```python
from build123d import *

# Parameters (mm, degrees)
SKETCH1_W               = 89.8
SKETCH1_H               = 61.4
BOSS_EXTRUDE1_DEPTH     = 6.9
SKETCH2_R               = 2
CUT_EXTRUDE1_DEPTH      = 4
SKETCH3_W               = 97
SKETCH3_H               = 70.6
BOSS_EXTRUDE2_DEPTH     = 5
SKETCH5_W               = 10.4
SKETCH5_H               = 6.9
SKETCH5_W_2             = 3.4
BOSS_EXTRUDE3_DEPTH     = 1.8
BOSS_EXTRUDE4_START     = 1.8
SKETCH5_3_W             = 10.4
SKETCH5_3_H             = 6.9
SKETCH5_3_H_2           = 27.6
SKETCH5_3_W_2           = 3.4
BOSS_EXTRUDE4_DEPTH     = 1
BOSS_EXTRUDE6_START     = -89.8
SKETCH5_5_W             = 3.4
SKETCH5_5_H             = 6.9
SKETCH5_5_W_2           = 10.4
BOSS_EXTRUDE6_DEPTH     = 1.8
BOSS_EXTRUDE7_START     = -91.6
SKETCH5_7_W             = 3.4
SKETCH5_7_H             = 6.9
SKETCH5_7_H_2           = 27.6
SKETCH5_7_W_2           = 10.4
BOSS_EXTRUDE7_DEPTH     = 1
CUT_EXTRUDE2_DEPTH      = 120.754123102
CUT_EXTRUDE2_DEPTH_BACK = 120.754123102
SKETCH6_R               = 3.2
BOSS_EXTRUDE9_START     = -24.4
BOSS_EXTRUDE9_DEPTH     = 23.4
BOSS_EXTRUDE10_START    = -92.4
SKETCH7_4_W             = 10
SKETCH7_4_H             = 7.6
SKETCH7_4_W_2           = 4
SKETCH7_4_H_2           = 7.2
BOSS_EXTRUDE10_DEPTH    = 23.4
SKETCH9_R               = 2
CUT_EXTRUDE3_DEPTH      = 4
MIRROR4_COPY_1_SKETCH_R = 2
MIRROR4_COPY_1_DEPTH    = 4
FILLET1_R               = 5
FILLET2_R               = 5
SKETCH12_R              = 2
CUT_EXTRUDE6_DEPTH      = 4


with BuildPart() as part:
    # Sketch1 → Boss-Extrude1 (new body)
    with BuildSketch(Plane(origin=(0, 0, 0), x_dir=(1, 0, 0), z_dir=(0, 1, 0))):
        with Locations((45.3, -31.1)):
            Rectangle(SKETCH1_W, SKETCH1_H)
        Polygon((81.1, 0), (81.1, 3.6), (9.5, 3.6), (9.5, 0), (9.5, -0.4), (81.1, -0.4), align=None)
    extrude(amount=BOSS_EXTRUDE1_DEPTH)

    # Sketch2 → Cut-Extrude1 (cut)
    with BuildSketch(Plane(origin=(90.2, 0, 0), x_dir=(0, 0, -1), z_dir=(1, 0, 0))):
        with Locations((-3.45, 3.45)):
            Circle(SKETCH2_R)
    cut_extrude1 = extrude(amount=-CUT_EXTRUDE1_DEPTH, mode=Mode.SUBTRACT)

    # Mirror1: Cut-Extrude1 across plane
    add(cut_extrude1.mirror(Plane(origin=(45.3, 0, 0), x_dir=(0, 0, 1), z_dir=(1, 0, 0))), mode=Mode.SUBTRACT)

    # Sketch3 → Boss-Extrude2 (add)
    with BuildSketch(Plane(origin=(0, 0, 0), x_dir=(1, 0, 0), z_dir=(0, 1, 0))):
        with Locations((45.3, -30.1)):
            Rectangle(SKETCH3_W, SKETCH3_H)
    extrude(amount=-BOSS_EXTRUDE2_DEPTH)

    # Sketch5 → Boss-Extrude3 (add)
    with BuildSketch(Plane.ZY.offset(-0.4)):
        with Locations((30.1, 3.45)):
            Rectangle(SKETCH5_W, SKETCH5_H)
        with Locations((23.2, 3.45)):
            Rectangle(SKETCH5_W_2, SKETCH5_H)
        with Locations((37, 3.45)):
            Rectangle(SKETCH5_W_2, SKETCH5_H)
    extrude(amount=BOSS_EXTRUDE3_DEPTH)

    # Sketch5<3> → Boss-Extrude4 (add)
    with BuildSketch(Plane.ZY.offset(-0.4).offset(BOSS_EXTRUDE4_START)):
        with Locations((30.1, 3.45)):
            Rectangle(SKETCH5_3_W, SKETCH5_3_H)
        with Locations((30.1, 20.7)):
            Rectangle(SKETCH5_3_W, SKETCH5_3_H_2)
        with Locations((23.2, 20.7)):
            Rectangle(SKETCH5_3_W_2, SKETCH5_3_H_2)
        with Locations((23.2, 3.45)):
            Rectangle(SKETCH5_3_W_2, SKETCH5_3_H)
        with Locations((37, 3.45)):
            Rectangle(SKETCH5_3_W_2, SKETCH5_3_H)
        with Locations((37, 20.7)):
            Rectangle(SKETCH5_3_W_2, SKETCH5_3_H_2)
    extrude(amount=-BOSS_EXTRUDE4_DEPTH)

    # Sketch5<5> → Boss-Extrude6 (add)
    with BuildSketch(Plane.ZY.offset(-0.4).offset(BOSS_EXTRUDE6_START)):
        with Locations((23.2, 3.45)):
            Rectangle(SKETCH5_5_W, SKETCH5_5_H)
        with Locations((37, 3.45)):
            Rectangle(SKETCH5_5_W, SKETCH5_5_H)
        with Locations((30.1, 3.45)):
            Rectangle(SKETCH5_5_W_2, SKETCH5_5_H)
    extrude(amount=-BOSS_EXTRUDE6_DEPTH)

    # Sketch5<7> → Boss-Extrude7 (add)
    with BuildSketch(Plane.ZY.offset(-0.4).offset(BOSS_EXTRUDE7_START)):
        with Locations((37, 3.45)):
            Rectangle(SKETCH5_7_W, SKETCH5_7_H)
        with Locations((37, 20.7)):
            Rectangle(SKETCH5_7_W, SKETCH5_7_H_2)
        with Locations((30.1, 20.7)):
            Rectangle(SKETCH5_7_W_2, SKETCH5_7_H_2)
        with Locations((23.2, 20.7)):
            Rectangle(SKETCH5_7_W, SKETCH5_7_H_2)
        with Locations((23.2, 3.45)):
            Rectangle(SKETCH5_7_W, SKETCH5_7_H)
        with Locations((30.1, 3.45)):
            Rectangle(SKETCH5_7_W_2, SKETCH5_7_H)
    extrude(amount=BOSS_EXTRUDE7_DEPTH)

    # Sketch6 → Cut-Extrude2 (cut, two sides: drawn at the far end of the back side and taken through both)
    with BuildSketch(Plane(origin=(-0.4, 0, 0), x_dir=(0, 0, -1), z_dir=(1, 0, 0)).offset(-CUT_EXTRUDE2_DEPTH_BACK)):
        with Locations((-30.1, 20.9)):
            Circle(SKETCH6_R)
    extrude(amount=CUT_EXTRUDE2_DEPTH + CUT_EXTRUDE2_DEPTH_BACK, mode=Mode.SUBTRACT)

    # Sketch7 → Boss-Extrude9 (add)
    with BuildSketch(Plane(origin=(92, 0, 0), x_dir=(0, 0, -1), z_dir=(1, 0, 0)).offset(BOSS_EXTRUDE9_START)):
        Polygon((-38.7, 34.5), (-38.7, 6.9), (-24.7, 6.9), (-24.7, 14.5), (-34.7, 14.5), (-34.7, 27.3), (-24.7, 27.3), (-24.7, 34.5), align=None)
    extrude(amount=BOSS_EXTRUDE9_DEPTH)

    # Sketch7<4> → Boss-Extrude10 (add)
    with BuildSketch(Plane(origin=(92, 0, 0), x_dir=(0, 0, -1), z_dir=(1, 0, 0)).offset(BOSS_EXTRUDE10_START)):
        with Locations((-29.7, 10.7)):
            Rectangle(SKETCH7_4_W, SKETCH7_4_H)
        with Locations((-36.7, 10.7)):
            Rectangle(SKETCH7_4_W_2, SKETCH7_4_H)
        with Locations((-36.7, 30.9)):
            Rectangle(SKETCH7_4_W_2, SKETCH7_4_H_2)
        with Locations((-29.7, 30.9)):
            Rectangle(SKETCH7_4_W, SKETCH7_4_H_2)
        Polygon((-38.7, 27.3), (-38.7, 20.9), (-38.7, 14.5), (-34.7, 14.5), (-34.7, 27.3), align=None)
    extrude(amount=BOSS_EXTRUDE10_DEPTH)

    # Sketch9 → Cut-Extrude3 (cut)
    with BuildSketch(Plane(origin=(0, 0, 24.7), x_dir=(-1, 0, 0), z_dir=(0, 0, -1))):
        with Locations(Location((-85.15, 30.9, 0), (0, 0, 90))):
            Circle(SKETCH9_R)
        with Locations(Location((-73.45, 30.9, 0), (0, 0, 270))):
            Circle(SKETCH9_R)
    cut_extrude3 = extrude(amount=-CUT_EXTRUDE3_DEPTH, mode=Mode.SUBTRACT)

    # Mirror3: Cut-Extrude3 across plane
    add(cut_extrude3.mirror(Plane(origin=(45.3, 0, 0), x_dir=(0, 0, 1), z_dir=(1, 0, 0))), mode=Mode.SUBTRACT)

    # Mirror4: Cut-Extrude3 across plane
    add(cut_extrude3.mirror(Plane.ZX.offset(20.7)), mode=Mode.SUBTRACT)

    # Mirror4 copy 1 sketch → Mirror4 copy 1 (cut)
    with BuildSketch(Plane(origin=(90.6, 41.4, 24.7), x_dir=(1, 0, 0), z_dir=(0, 0, -1))):
        with Locations(Location((-85.15, 30.9, 0), (0, 0, 90))):
            Circle(MIRROR4_COPY_1_SKETCH_R)
        with Locations(Location((-73.45, 30.9, 0), (0, 0, 270))):
            Circle(MIRROR4_COPY_1_SKETCH_R)
    extrude(amount=-MIRROR4_COPY_1_DEPTH, mode=Mode.SUBTRACT)

    # Fillet1
    fillet1_edges = [part.edges().sort_by_distance(p)[0] for p in [
        (93.8, -2.5, -5.2),
        (93.8, -2.5, 65.4),
        (-3.2, -2.5, 65.4),
        (-3.2, -2.5, -5.2),
    ]]
    fillet(fillet1_edges, radius=FILLET1_R)

    # Fillet2
    fillet2_edges = [part.edges().sort_by_distance(p)[0] for p in [
        (92.335533906, -5, 63.935533906),
        (93.8, -5, 30.1),
        (92.335533906, -5, -3.735533906),
        (45.3, -5, -5.2),
        (-1.735533906, -5, -3.735533906),
        (-3.2, -5, 30.1),
        (-1.735533906, -5, 63.935533906),
        (45.3, -5, 65.4),
    ]]
    fillet(fillet2_edges, radius=FILLET2_R - 0.0001)  # a hair under: the kernel refuses the full size

    # Sketch12 → Cut-Extrude6 (cut)
    with BuildSketch(Plane(origin=(90.2, 0, 0), x_dir=(0, 0, -1), z_dir=(1, 0, 0))):
        with Locations((-56.75, 3.45)):
            Circle(SKETCH12_R)
    cut_extrude6 = extrude(amount=-CUT_EXTRUDE6_DEPTH, mode=Mode.SUBTRACT)

    # Mirror5: Cut-Extrude6 across plane
    add(cut_extrude6.mirror(Plane(origin=(45.3, 0, 0), x_dir=(0, 0, 1), z_dir=(1, 0, 0))), mode=Mode.SUBTRACT)


solid = part.part
```
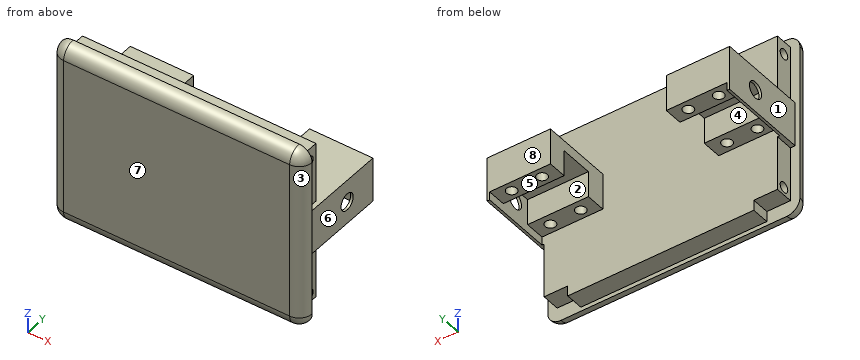
Here's how the part is built. I have some questions about the finished solid (model axes, mm). Face numbers are marked on the shaded views. A direction names the side the tool comes from. Coordinates: 2 decimals unless noted, no trailing zeros. Loops run counter-clockwise (first coordinate to the right, second up) from the corner with the lowest first, then second, coordinate; pieces in that order, holes last. Notation, with made-up numbers: (-11.75, 60.25) - (23.25, 60.25) arc R13 cw to (23.25, 72.25) - close; hole circle Ø2 at (-3, -32). An arc over 180 degrees is marked (long way). Return JSON: item names as keys, results as strings. Group by question number.
Item 1: Will these pins go through, and if not, where does the flat tip stop? P1, Ø10, axis at y = 8.5, z = 9.5, coming from the -X side; P2, Ø3, axis at x = 85.15, y = 10.5, coming from the -Z side; P3, Ø6, axis at x = 23.5, y = 24, coming from the -Z side.
Item 2: If we section it at B-B on y = 20.9: Write out the boundary of the cut face in (x, z), and give its area (3 significant figures).
Item 3: If we section it at A-A on z = 30.1: State how many separate pieces and enclosed holes the cut face has, and give its area (3 significant figures).
Item 4: We'd pull the mould along Y, two halves only. Please class the marked faces 1, 2 and 3: +Y half, -Y half, draft (parallel to the pull), parting line (faces both ways), or undercut.
Item 5: On a 3-axis mill with a long thin cutter (end or side, diameter ignored), from which of +Z, -Z, +X, -X, +Y, -Y can I reach the whole of each face in a straight line? I mean the marked faces 4, 5, 6, 7 and 8. Say none if no direction works.
Item 6: If we section it at D-D on y = 10.5: Write out the boundary of the cut face in (x, z), and give its area (3 significant figures).
Item 7: I need wall thicknesses on line 1 (Y direction, x = 17, z = 26); line 2 (Y direction, x = 87.5, z = 27); line 3 (X direction, y = 30.9, z = 27.8). Which ranges of each line are inside material? Lowest first, please. Write a range as from..to.
Calculated:
{
 "1": {"P1": "stops at x = 0.4", "P2": "stops at z = 28.7", "P3": "stops at z = 34.7"},
 "2": {"outline": "(-1.4, 21.5) - (-0.4, 21.5) - (-0.4, 26.9) - (-1.4, 26.9) - close; (-1.4, 33.3) - (-0.4, 33.3) - (-0.4, 34.7) - (23, 34.7) - (23, 38.7) - (-1.4, 38.7) - close; (67.6, 34.7) - (91, 34.7) - (91, 33.3) - (92, 33.3) - (92, 38.7) - (67.6, 38.7) - close; (91, 21.5) - (92, 21.5) - (92, 26.9) - (91, 26.9) - close", "area": "209 mm^2"},
 "3": {"separate pieces": "3", "enclosed holes": "0", "area": "1,850 mm^2"},
 "4": {"face 1": "draft", "face 2": "undercut", "face 3": "-Y half"},
 "5": {"face 4": "-Z", "face 5": "-Z, +Y", "face 6": "+Z, -Z, +X, +Y", "face 7": "+Z, -Z, +X, -X, -Y", "face 8": "+Z, -Z, +X, -X, +Y"},
 "6": {"outline": "(-1.4, 21.5) - (-0.4, 21.5) - (-0.4, 24.7) - (3.45, 24.7) - (3.45, 28.7) - (7.45, 28.7) - (7.45, 24.7) - (15.15, 24.7) - (15.15, 28.7) - (19.15, 28.7) - (19.15, 24.7) - (23, 24.7) - (23, 38.7) - (-1.4, 38.7) - close; (67.6, 24.7) - (71.45, 24.7) - (71.45, 28.7) - (75.45, 28.7) - (75.45, 24.7) - (83.15, 24.7) - (83.15, 28.7) - (87.15, 28.7) - (87.15, 24.7) - (91, 24.7) - (91, 21.5) - (92, 21.5) - (92, 38.7) - (67.6, 38.7) - close", "area": "626 mm^2"},
 "7": {"line 1": "y = -5..8.51, 12.49..14.5, 27.3..28.91, 32.89..34.5", "line 2": "y = -5..14.5, 27.3..34.5", "line 3": "x = -1.4..3.45, 7.45..15.15, 19.15..23, 67.6..71.45, 75.45..83.15, 87.15..92"}
}
